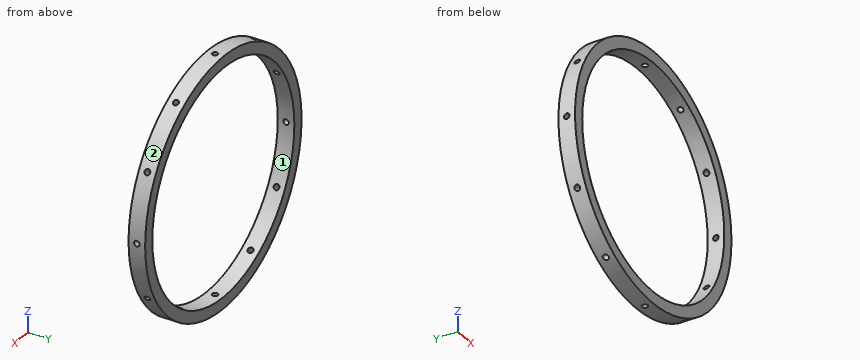
from build123d import *

# Parameters (mm, degrees)
SKETCH1_R           = 95.25
SKETCH1_R_2         = 86.487
BOSS_EXTRUDE1_DEPTH = 12.7
SKETCH3_R           = 2.1463
CUT_EXTRUDE2_DEPTH  = 254
CIRPATTERN1_COUNT   = 12


with BuildPart() as part:
    # Sketch1 → Boss-Extrude1 (new body)
    with BuildSketch(Plane(origin=(0, 0, 0), x_dir=(1, 0, 0), z_dir=(0, 1, 0))):
        Circle(SKETCH1_R)
        Circle(SKETCH1_R_2, mode=Mode.SUBTRACT)
    extrude(amount=BOSS_EXTRUDE1_DEPTH)

    # Sketch3 → Cut-Extrude2 (cut)
    with BuildSketch(Plane.XY):
        with Locations((0, 6.35)):
            Circle(SKETCH3_R)
    cut_extrude2 = extrude(amount=-CUT_EXTRUDE2_DEPTH, mode=Mode.SUBTRACT)

    # CirPattern1: Cut-Extrude2 ×12 about axis
    cirpattern1_axis = Axis((0, 12.7, 0), (0, 1, 0))
    for i in range(1, CIRPATTERN1_COUNT):
        add(cut_extrude2.rotate(cirpattern1_axis, i * 360 / CIRPATTERN1_COUNT), mode=Mode.SUBTRACT)


solid = part.part
Build history of the part. All positions in model axes, mm. Face numbers are marked on the shaded views. Coordinates: 2 decimals unless noted, no trailing zeros. Order: outer loops, then holes, each group sorted by start corner. A loop starts at its lowest first (then second) coordinate and runs counter-clockwise, first axis right, second up. Notation, with made-up numbers: M 79.25,47 L 90.25,47 A21 ccw 90.25,69 Z; hole C 15,39.5 d10. An arc over 180 degrees is marked long. One line per question, with ' | ' between items. Start each with the question number.
Q1. Saw through at B-B (z = 66). List the corners of the cut face in (x, y).
Q2. Saw through at A-A (x = 32.5). List the corners of the cut face in (y, z), then the cut area to 3 significant figures.
Q3. Flat gauge pins, fed straight in: pin 1 Ø4 at (x, y) = (0, 6.35) entering from -Z; pin 2 Ø1 at (x, y) = (-29, 6) entering from +Z; pin 3 Ø6 at (x, y) = (61, 6.5) entering from -Z (3 decimals); pin 4 Ø3 at (x, y) = (7.5, 9.5) entering from +Z. Where does each tip first touch, or does it go through?
Q4. Probe L1, parallel to Y at x = -93.25, z = 0; L2, parallel to Z at x = 24.5, y = 4.75; L3, parallel to Z at x = -73.5, y = 10. List the from-to ranges inside material, lowest first. Write a range as from..to.
Q5. Two-plate mould, pull along X, no slides. Class the marked faces 1 and 2: +X half, -X half, draft (parallel to the pull), parting line (faces both ways), or undercut.
Q6. Saw through at C-C (y = 6.35). Count the separate pieces of the cut face and the enclosed holes in it, then the cut area to 3 significant figures.
Check values:
1) outline: M -68.68,0 L -55.89,0 L -55.89,12.7 L -68.68,12.7 Z; M 55.89,0 L 68.68,0 L 68.68,12.7 L 55.89,12.7 Z
2) outline: M 0,-89.53 L 12.7,-89.53 L 12.7,-80.15 L 0,-80.15 Z; M 0,80.15 L 12.7,80.15 L 12.7,89.53 L 0,89.53 Z | area: 238 mm2
3) pin 1: passes through | pin 2: stops at z = 90.89 | pin 3: stops at z = -75.555 | pin 4: stops at z = 95.06
4) L1: y = 0..4.2, 8.5..12.7 | L2: z = -92.05..-82.94, 82.94..92.05 | L3: z = -60.58..-45.58, 45.58..60.58
5) face 1: undercut | face 2: parting line
6) separate pieces: 12 | enclosed holes: 0 | area: 4,550 mm2
